from build123d import *

# Parameters (mm, degrees)
SKETCH_2_W          = 11.343097154
SKETCH_2_H          = 1.6
CUT_EXTRUDE_1_DEPTH = 1.8


with BuildPart() as part:
    # 스케치1 → 회전1 (revolve)
    with BuildSketch(Plane(origin=(0, 0, 0), x_dir=(0, 0, -1), z_dir=(1, 0, 0))):
        Polygon((0, 0), (0, 4.55), (3.3, 4.55), (3.3, 3), (11.2, 3), (11.2, 0), align=None)
    revolve(axis=Axis((0, 0, -11.2), (0, 0, 1)))

    # 스케치2 → 컷-돌출1 (cut)
    with BuildSketch(Plane.XY):
        with Locations((-0.136663821, 0)):
            Rectangle(SKETCH_2_W, SKETCH_2_H)
    extrude(amount=-CUT_EXTRUDE_1_DEPTH, mode=Mode.SUBTRACT)


solid = part.part
Verification items for the finished model (mm, model axes). A direction names the side the tool comes from. Round coordinates to 2 decimals unless told otherwise and drop trailing zeros. Order: outer loops, then holes, each group sorted by start corner. A loop starts at its lowest first (then second) coordinate and runs counter-clockwise, first axis right, second up.
1. Access from +Z, -Z, +X, -X, +Y, -Y to the whole of each face (thin tool, end or side, straight path). Record for faces 4 (the flat face through (1, 3, -3.3)), 5 (the flat face through (0, -0.8, -1)), 6 (the flat face through (0, 2, 0)).
Final values:
face 4: -Z
face 5: +Z, +X, -X
face 6: +Z, +X, -X, +Y, -Y
2. Section check B-B on x = 0. Record the cut outline in (y, z), then the cut area to 4 significant figures.
Final values:
outline: (-4.55, -3.3) - (-3, -3.3) - (-3, -11.2) - (3, -11.2) - (3, -3.3) - (4.55, -3.3) - (4.55, 0) - (0.8, 0) - (0.8, -1.8) - (-0.8, -1.8) - (-0.8, 0) - (-4.55, 0) - close
area: 74.55 mm2
3. Section check C-C on z = -7.25. Record the cut outline in (x, y).
Final values:
outline: circle Ø6 at (0, 0)
4. Section check A-A on y = 0. Record the cut outline in (x, z), then the cut area to 4 significant figures.
Final values:
outline: (-4.55, -3.3) - (-3, -3.3) - (-3, -11.2) - (3, -11.2) - (3, -3.3) - (4.55, -3.3) - (4.55, -1.8) - (-4.55, -1.8) - close
area: 61.05 mm2
5. Section check D-D on y = -1.25. Record the cut outline in (x, z), then the cut area to 3 significant figures.
Final values:
outline: (-4.37, -3.3) - (-2.73, -3.3) - (-2.73, -11.2) - (2.73, -11.2) - (2.73, -3.3) - (4.37, -3.3) - (4.37, 0) - (-4.37, 0) - close
area: 72.0 mm2
6. Thickness scan on L1, parallel to Z at x = -3, y = -1.5; L2, parallel to Y at x = 1, z = -1.5; L3, parallel to Y at x = -1.5, z = -0.75. Record the ranges inside material, lowest first.
Final values:
L1: z = -3.3 to 0
L2: y = -4.44 to -0.8, 0.8 to 4.44
L3: y = -4.3 to -0.8, 0.8 to 4.3
7. Release check for a two-part mould opening along Y. For faces 1 (the flat face through (0, 0, -1.8)), 2 (the flat face through (0, 0, -11.2)), 3 (the cylindrical face through (0, -3, -7)) record: +Y half, -Y half, draft (parallel to the pull), parting line (faces both ways), or undercut.
Final values:
face 1: undercut
face 2: draft
face 3: parting line
8. Go/stop test with flat-tipped pins: P1, Ø3, axis at x = 1.5, z = -5.5, coming from the +Y side; P2, Ø0.8, axis at x = 0.5, y = 0, coming from the +Z side; P3, Ø1, axis at x = 0.5, z = -8.5, coming from the -Y side; P4, Ø3, axis at x = 0.5, y = -3, coming from the -Z side. Record where each tip stops, or that it passes through.
Final values:
P1: stops at y = 3
P2: stops at z = -1.8
P3: stops at y = -3
P4: stops at z = -11.2
